Could you check a few things on this drawing? It's one solid part, dimensions in mm from its lowest x, y, z. A direction names the side the tool comes from. Coordinates: 2 decimals unless noted, no trailing zeros. Loops run counter-clockwise (first coordinate to the right, second up) from the corner with the lowest first, then second, coordinate; pieces in that order, holes last.
1) Will these pins go through, and if not, where does the flat tip stop? P1, Ø3.5, axis at x = 8, z = 10, coming from the +Y side; P2, Ø1.5, axis at x = 40.5, z = 15, coming from the +Y side; P3, Ø4, axis at x = 48.24, y = 9.25, coming from the -Z side; P4, Ø1.6, axis at y = 9, z = 19, coming from the +X side.
2) Imagine slicing it at B-B on y = 9.25. Please give me the cut outline in (x, z), plus the area to 3 significant figures.
3) For the marked faces 1 and 2, which set-ups out of +Z, -Z, +X, -X, +Y, -Y let a thin tool reach every point of the face, with its end or its side?
4) Imagine slicing it at D-D on x = 22.5. Please give me the cut outline in (y, z), plus the area to 3 significant figures.
5) If I drill on line 1 along X through (y, z) = (0.8, 10); line 2 along Z through (x, y) = (96, 1.65); line 3 along Y through (x, z) = (92, 18), over which ranges is the centre line in solid material (lowest first)?
6) Imagine slicing it at C-C on x = 96. Please give me the cut outline in (y, z), plus the area to 3 significant figures.
7) Imagine slicing it at A-A on z = 10. Please give me the cut outline in (x, y).
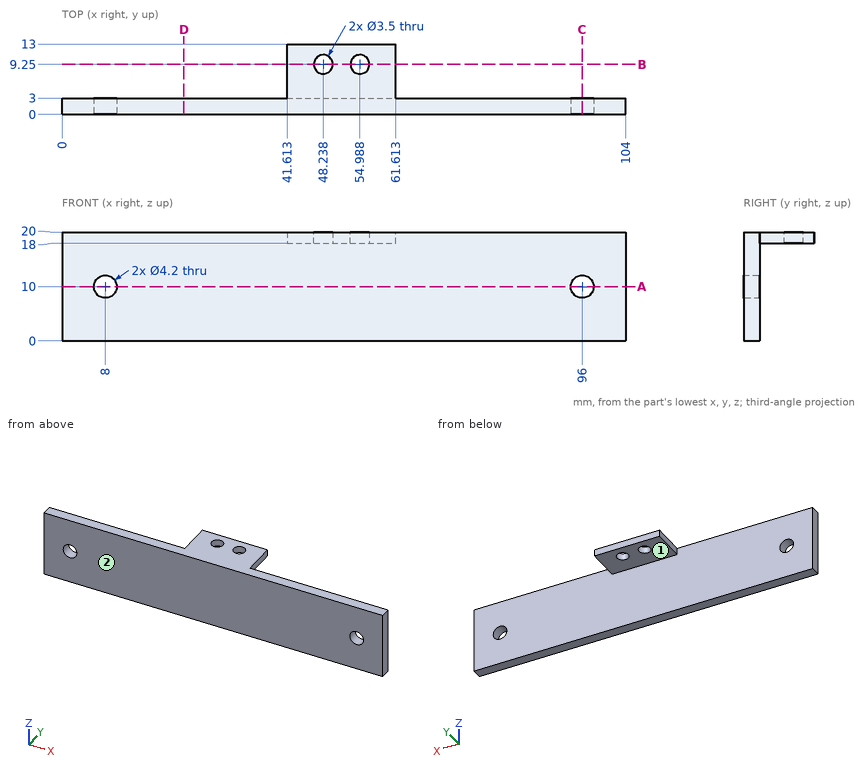
Filled in:
1. P1: passes through
1. P2: stops at y = 3
1. P3: stops at z = 18
1. P4: stops at x = 61.61
2. outline: (41.61, 18) - (46.49, 18) - (46.49, 20) - (41.61, 20) - close; (49.99, 18) - (53.24, 18) - (53.24, 20) - (49.99, 20) - close; (56.74, 18) - (61.61, 18) - (61.61, 20) - (56.74, 20) - close
2. area: 26.0 mm2
3. face 1: -Z, +X, -X, +Y
3. face 2: +Z, -Z, +X, -X, -Y
4. outline: (0, 0) - (3, 0) - (3, 20) - (0, 20) - close
4. area: 60.0 mm2
5. line 1: x = 0 to 5.9, 10.1 to 93.9, 98.1 to 104
5. line 2: z = 0 to 7.9, 12.1 to 20
5. line 3: y = 0 to 3
6. outline: (0, 0) - (3, 0) - (3, 7.9) - (0, 7.9) - close; (0, 12.1) - (3, 12.1) - (3, 20) - (0, 20) - close
6. area: 47.4 mm2
7. outline: (0, 0) - (5.9, 0) - (5.9, 3) - (0, 3) - close; (10.1, 0) - (93.9, 0) - (93.9, 3) - (10.1, 3) - close; (98.1, 0) - (104, 0) - (104, 3) - (98.1, 3) - close
